from build123d import *

# Parameters (mm, degrees)
SKETCH1_W               = 82
SKETCH1_H               = 46
BOSS_EXTRUDE1_DEPTH     = 25
CUT_EXTRUDE1_REACH      = 70.629
SKETCH2_W               = 76
SKETCH2_H               = 40
CUT_EXTRUDE2_DEPTH      = 89.758098222
CUT_EXTRUDE2_DEPTH_BACK = 89.758098222
SKETCH4_W               = 50
SKETCH4_H               = 3
BOSS_EXTRUDE2_DEPTH     = 71
CUT_EXTRUDE3_REACH      = 124.548
SKETCH5_R               = 1.75
SKETCH7_W               = 16
SKETCH7_H               = 3
BOSS_EXTRUDE4_DEPTH     = 71
SKETCH8_W               = 50
SKETCH8_H               = 46
BOSS_EXTRUDE5_DEPTH     = 3
CUT_EXTRUDE4_DEPTH      = 127.356638132
CUT_EXTRUDE4_DEPTH_BACK = 3
CUT_EXTRUDE5_REACH      = 128.357
SKETCH10_W              = 11
SKETCH10_H              = 5
CUT_EXTRUDE6_REACH      = 128.357
SKETCH11_R              = 1.5
SKETCH12_R              = 15
BOSS_EXTRUDE6_DEPTH     = 30
SKETCH13_R              = 12.5
CUT_EXTRUDE7_DEPTH      = 190.076704012
SKETCH14_W              = 2
SKETCH14_H              = 10.8
SKETCH14_H_2            = 13
BOSS_EXTRUDE7_DEPTH     = 68
CUT_EXTRUDE8_REACH      = 189.343
SKETCH15_R              = 2


with BuildPart() as part:
    # Sketch1 → Boss-Extrude1 (new, symmetric)
    with BuildSketch(Plane.XY):
        Rectangle(SKETCH1_W, SKETCH1_H)
    extrude(amount=BOSS_EXTRUDE1_DEPTH, both=True)

    # Sketch2 → Cut-Extrude1 (cut, up to next)
    with BuildSketch(Plane.XY.offset(25), mode=Mode.PRIVATE) as cut_extrude1_sk1:
        Rectangle(SKETCH2_W, SKETCH2_H)
    cut_extrude1_tool1 = extrude(cut_extrude1_sk1.sketch, amount=-CUT_EXTRUDE1_REACH, mode=Mode.PRIVATE) & part.part
    add(cut_extrude1_tool1.solids().sort_by_distance((0, 0, 25))[0], mode=Mode.SUBTRACT)

    # Sketch3 → Cut-Extrude2 (cut, two sides: drawn at the far end of the back side and taken through both)
    with BuildSketch(Plane.ZY.offset(41).offset(-CUT_EXTRUDE2_DEPTH_BACK)):
        Polygon((-18, 16), (-18, 20), (18, 20), (18, 16), (22, 16), (22, -16), (18, -16), (18, -20), (-18, -20), (-18, -16), (-22, -16), (-22, 16), align=None)
    extrude(amount=CUT_EXTRUDE2_DEPTH + CUT_EXTRUDE2_DEPTH_BACK, mode=Mode.SUBTRACT)

    # Sketch4 → Boss-Extrude2 (add)
    with BuildSketch(Plane(origin=(41, 0, 0), x_dir=(0, 0, -1), z_dir=(1, 0, 0))):
        with Locations((0, -21.5)):
            Rectangle(SKETCH4_W, SKETCH4_H)
    boss_extrude2 = extrude(amount=BOSS_EXTRUDE2_DEPTH)

    # Sketch5 → Cut-Extrude3 (cut, up to next)
    with BuildSketch(Plane(origin=(0, -20, 0), x_dir=(1, 0, 0), z_dir=(0, 1, 0)), mode=Mode.PRIVATE) as cut_extrude3_sk1:
        with Locations(Location((103.1, 20.1, 0), (0, 0, 270))):
            Circle(SKETCH5_R)
    cut_extrude3_tool1 = extrude(cut_extrude3_sk1.sketch, amount=-CUT_EXTRUDE3_REACH, mode=Mode.PRIVATE) & part.part
    # Sketch5 → Cut-Extrude3 (cut, up to next)
    with BuildSketch(Plane(origin=(0, -20, 0), x_dir=(1, 0, 0), z_dir=(0, 1, 0)), mode=Mode.PRIVATE) as cut_extrude3_sk2:
        with Locations(Location((103, -20, 0), (0, 0, 270))):
            Circle(SKETCH5_R)
    cut_extrude3_tool2 = extrude(cut_extrude3_sk2.sketch, amount=-CUT_EXTRUDE3_REACH, mode=Mode.PRIVATE) & part.part
    # Sketch5 → Cut-Extrude3 (cut, up to next)
    with BuildSketch(Plane(origin=(0, -20, 0), x_dir=(1, 0, 0), z_dir=(0, 1, 0)), mode=Mode.PRIVATE) as cut_extrude3_sk3:
        with Locations(Location((50, 20.1, 0), (0, 0, 270))):
            Circle(SKETCH5_R)
    cut_extrude3_tool3 = extrude(cut_extrude3_sk3.sketch, amount=-CUT_EXTRUDE3_REACH, mode=Mode.PRIVATE) & part.part
    # Sketch5 → Cut-Extrude3 (cut, up to next)
    with BuildSketch(Plane(origin=(0, -20, 0), x_dir=(1, 0, 0), z_dir=(0, 1, 0)), mode=Mode.PRIVATE) as cut_extrude3_sk4:
        with Locations(Location((50, -20, 0), (0, 0, 270))):
            Circle(SKETCH5_R)
    cut_extrude3_tool4 = extrude(cut_extrude3_sk4.sketch, amount=-CUT_EXTRUDE3_REACH, mode=Mode.PRIVATE) & part.part
    cut_extrude3_1 = cut_extrude3_tool1.solids().sort_by_distance((103.1, -20, -20.1))[0]
    add(cut_extrude3_1, mode=Mode.SUBTRACT)
    cut_extrude3_2 = cut_extrude3_tool2.solids().sort_by_distance((103, -20, 20))[0]
    add(cut_extrude3_2, mode=Mode.SUBTRACT)
    cut_extrude3_3 = cut_extrude3_tool3.solids().sort_by_distance((50, -20, -20.1))[0]
    add(cut_extrude3_3, mode=Mode.SUBTRACT)
    cut_extrude3_4 = cut_extrude3_tool4.solids().sort_by_distance((50, -20, 20))[0]
    add(cut_extrude3_4, mode=Mode.SUBTRACT)
    cut_extrude3 = cut_extrude3_1 + cut_extrude3_2 + cut_extrude3_3 + cut_extrude3_4  # Cut-Extrude3 as one shape, for the pattern or mirror that repeats it

    # Sketch7 → Boss-Extrude4 (add)
    with BuildSketch(Plane(origin=(41, 0, 0), x_dir=(0, 0, -1), z_dir=(1, 0, 0))):
        with Locations((0, 21.5)):
            Rectangle(SKETCH7_W, SKETCH7_H)
    boss_extrude4 = extrude(amount=BOSS_EXTRUDE4_DEPTH)

    # Sketch8 → Boss-Extrude5 (add)
    with BuildSketch(Plane(origin=(112, 0, 0), x_dir=(0, 0, -1), z_dir=(1, 0, 0))):
        Rectangle(SKETCH8_W, SKETCH8_H)
    extrude(amount=BOSS_EXTRUDE5_DEPTH)

    # Sketch9 → Cut-Extrude4 (cut, two sides: drawn at the far end of the back side and taken through both)
    with BuildSketch(Plane(origin=(0, 23, 0), x_dir=(1, 0, 0), z_dir=(0, 1, 0)).offset(-CUT_EXTRUDE4_DEPTH_BACK)):
        Polygon((105, -317.365996733), (105, -8), (105, -3), (94, -3), (94, -8), (94, -317.365996733), (94, -936.097990199), (105, -936.097990199), align=None)
    extrude(amount=CUT_EXTRUDE4_DEPTH + CUT_EXTRUDE4_DEPTH_BACK, mode=Mode.SUBTRACT)

    # Sketch10 → Cut-Extrude5 (cut, up to next)
    with BuildSketch(Plane(origin=(0, 23, 0), x_dir=(1, 0, 0), z_dir=(0, 1, 0)), mode=Mode.PRIVATE) as cut_extrude5_sk1:
        with Locations((53.5, -5.5)):
            Rectangle(SKETCH10_W, SKETCH10_H)
    cut_extrude5_tool1 = extrude(cut_extrude5_sk1.sketch, amount=-CUT_EXTRUDE5_REACH, mode=Mode.PRIVATE) & part.part
    add(cut_extrude5_tool1.solids().sort_by_distance((53.5, 23, 5.5))[0], mode=Mode.SUBTRACT)

    # Sketch11 → Cut-Extrude6 (cut, up to next)
    with BuildSketch(Plane(origin=(0, 23, 0), x_dir=(1, 0, 0), z_dir=(0, 1, 0)), mode=Mode.PRIVATE) as cut_extrude6_sk1:
        with Locations(Location((45.5, -5.5, 0), (0, 0, 270))):
            Circle(SKETCH11_R)
    cut_extrude6_tool1 = extrude(cut_extrude6_sk1.sketch, amount=-CUT_EXTRUDE6_REACH, mode=Mode.PRIVATE) & part.part
    # Sketch11 → Cut-Extrude6 (cut, up to next)
    with BuildSketch(Plane(origin=(0, 23, 0), x_dir=(1, 0, 0), z_dir=(0, 1, 0)), mode=Mode.PRIVATE) as cut_extrude6_sk2:
        with Locations(Location((61.5, -5.5, 0), (0, 0, 270))):
            Circle(SKETCH11_R)
    cut_extrude6_tool2 = extrude(cut_extrude6_sk2.sketch, amount=-CUT_EXTRUDE6_REACH, mode=Mode.PRIVATE) & part.part
    # Sketch11 → Cut-Extrude6 (cut, up to next)
    with BuildSketch(Plane(origin=(0, 23, 0), x_dir=(1, 0, 0), z_dir=(0, 1, 0)), mode=Mode.PRIVATE) as cut_extrude6_sk3:
        with Locations(Location((91.5, -5.5, 0), (0, 0, 270))):
            Circle(SKETCH11_R)
    cut_extrude6_tool3 = extrude(cut_extrude6_sk3.sketch, amount=-CUT_EXTRUDE6_REACH, mode=Mode.PRIVATE) & part.part
    # Sketch11 → Cut-Extrude6 (cut, up to next)
    with BuildSketch(Plane(origin=(0, 23, 0), x_dir=(1, 0, 0), z_dir=(0, 1, 0)), mode=Mode.PRIVATE) as cut_extrude6_sk4:
        with Locations(Location((107.5, -5.5, 0), (0, 0, 270))):
            Circle(SKETCH11_R)
    cut_extrude6_tool4 = extrude(cut_extrude6_sk4.sketch, amount=-CUT_EXTRUDE6_REACH, mode=Mode.PRIVATE) & part.part
    add(cut_extrude6_tool1.solids().sort_by_distance((45.5, 23, 5.5))[0], mode=Mode.SUBTRACT)
    add(cut_extrude6_tool2.solids().sort_by_distance((61.5, 23, 5.5))[0], mode=Mode.SUBTRACT)
    add(cut_extrude6_tool3.solids().sort_by_distance((91.5, 23, 5.5))[0], mode=Mode.SUBTRACT)
    add(cut_extrude6_tool4.solids().sort_by_distance((107.5, 23, 5.5))[0], mode=Mode.SUBTRACT)

    # Sketch12 → Boss-Extrude6 (add)
    with BuildSketch(Plane(origin=(115, 0, 0), x_dir=(0, 0, -1), z_dir=(1, 0, 0))):
        with Locations((10, 0)):
            Circle(SKETCH12_R)
    extrude(amount=BOSS_EXTRUDE6_DEPTH)

    # Sketch13 → Cut-Extrude7 (cut, through all)
    with BuildSketch(Plane(origin=(145, 0, 0), x_dir=(0, 0, -1), z_dir=(1, 0, 0))):
        with Locations((10, 0)):
            Circle(SKETCH13_R)
    extrude(amount=-CUT_EXTRUDE7_DEPTH, mode=Mode.SUBTRACT)

    # Sketch14 → Boss-Extrude7 (add)
    with BuildSketch(Plane(origin=(115, 0, 0), x_dir=(0, 0, -1), z_dir=(1, 0, 0))):
        with Locations((-3.7, 17.6)):
            Rectangle(SKETCH14_W, SKETCH14_H)
        with Locations((-3.7, -22.5)):
            Rectangle(SKETCH14_W, SKETCH14_H_2)
    extrude(amount=BOSS_EXTRUDE7_DEPTH)

    # Sketch15 → Cut-Extrude8 (cut, up to next)
    with BuildSketch(Plane(origin=(0, 0, 2.7), x_dir=(-1, 0, 0), z_dir=(0, 0, -1)), mode=Mode.PRIVATE) as cut_extrude8_sk1:
        with Locations(Location((-180, -24.8, 0), (0, 0, 90))):
            Circle(SKETCH15_R)
    cut_extrude8_tool1 = extrude(cut_extrude8_sk1.sketch, amount=-CUT_EXTRUDE8_REACH, mode=Mode.PRIVATE) & part.part
    # Sketch15 → Cut-Extrude8 (cut, up to next)
    with BuildSketch(Plane(origin=(0, 0, 2.7), x_dir=(-1, 0, 0), z_dir=(0, 0, -1)), mode=Mode.PRIVATE) as cut_extrude8_sk2:
        with Locations(Location((-160, -24.8, 0), (0, 0, 90))):
            Circle(SKETCH15_R)
    cut_extrude8_tool2 = extrude(cut_extrude8_sk2.sketch, amount=-CUT_EXTRUDE8_REACH, mode=Mode.PRIVATE) & part.part
    # Sketch15 → Cut-Extrude8 (cut, up to next)
    with BuildSketch(Plane(origin=(0, 0, 2.7), x_dir=(-1, 0, 0), z_dir=(0, 0, -1)), mode=Mode.PRIVATE) as cut_extrude8_sk3:
        with Locations(Location((-160, 17.2, 0), (0, 0, 90))):
            Circle(SKETCH15_R)
    cut_extrude8_tool3 = extrude(cut_extrude8_sk3.sketch, amount=-CUT_EXTRUDE8_REACH, mode=Mode.PRIVATE) & part.part
    # Sketch15 → Cut-Extrude8 (cut, up to next)
    with BuildSketch(Plane(origin=(0, 0, 2.7), x_dir=(-1, 0, 0), z_dir=(0, 0, -1)), mode=Mode.PRIVATE) as cut_extrude8_sk4:
        with Locations(Location((-180, 17.2, 0), (0, 0, 90))):
            Circle(SKETCH15_R)
    cut_extrude8_tool4 = extrude(cut_extrude8_sk4.sketch, amount=-CUT_EXTRUDE8_REACH, mode=Mode.PRIVATE) & part.part
    add(cut_extrude8_tool1.solids().sort_by_distance((180, -24.8, 2.7))[0], mode=Mode.SUBTRACT)
    add(cut_extrude8_tool2.solids().sort_by_distance((160, -24.8, 2.7))[0], mode=Mode.SUBTRACT)
    add(cut_extrude8_tool3.solids().sort_by_distance((160, 17.2, 2.7))[0], mode=Mode.SUBTRACT)
    add(cut_extrude8_tool4.solids().sort_by_distance((180, 17.2, 2.7))[0], mode=Mode.SUBTRACT)

    # Mirror1: Boss-Extrude2, Cut-Extrude3, Boss-Extrude4 across plane
    add(boss_extrude2.mirror(Plane(origin=(0, 0, 0), x_dir=(0, 0, 1), z_dir=(1, 0, 0))))
    add(cut_extrude3.mirror(Plane(origin=(0, 0, 0), x_dir=(0, 0, 1), z_dir=(1, 0, 0))), mode=Mode.SUBTRACT)
    add(boss_extrude4.mirror(Plane(origin=(0, 0, 0), x_dir=(0, 0, 1), z_dir=(1, 0, 0))))


solid = part.part
Design review of the part built by this model. Coordinates are the model's own, in mm. A direction names the side the tool comes from. Coordinates: 2 decimals unless noted, no trailing zeros. Loops run counter-clockwise (first coordinate to the right, second up) from the corner with the lowest first, then second, coordinate; pieces in that order, holes last. Notation, with made-up numbers: (14, 30.25) - (71, 30.25) arc R19 cw to (71, 35.25) - close; hole circle Ø5 at (43.25, -0.75). An arc over 180 degrees is marked (long way). Use CSV: the item, a comma, the result in double quotes. Start each with the question number.
1. Add section D-D on x = 77. Give the boundary of the cut face in (y, z), plus the area to 3 significant figures.
2. Add section A-A on x = 7. Give the boundary of the cut face in (y, z).
3. Mouldability with a two-part tool opening along X and no side actions: class faces 6 (the flat face through (41, 5, -23)), 7 (the flat face through (149, 18, 4.7)), 8 (the flat face through (-41, 4.6, 22.2)) as released by +X, released by -X, zero draft, split by the parting line, or undercut.
4. Clearance check with flat-ended pins moving along their axes: pin 1 (6 mm diameter, centred on x = 131.5, y = -13.5, fed in from +Z); pin 2 (4 mm diameter, centred on x = -8, z = -19.5, fed in from -Y); pin 3 (2 mm diameter, centred on y = -19, z = 10.5, fed in from +X); pin 4 (4 mm diameter, centred on x = 107.5, z = 5.5, fed in from +Y). State where each tip first meets the part, or that it passes through.
5. Add section C-C on y = 8. Give the boundary of the cut face in (x, z).
6. To check wall thickness, follow probe 1 along Y at (x, z) = (160, 3.75); probe 2 along X at (y, z) = (-20.65, -20.1); probe 3 along Z at (x, y) = (103, -22). State the ranges of each line that lie inside material, in increasing order.
7. For faces 1 (the flat face through (-41, 5, -23)), 2 (the flat face through (149, -23, 4.7)), 3 (the flat face through (-6, -21, 25)), 4 (the flat face through (41, 4.6, 22.2)), 5 (the flat face through (38, 0, -23)), list the 3-axis set-ups (+Z, -Z, +X, -X, +Y, -Y) from which the entire face can be reached by the end or side of a thin tool; tool diameter is ignored.
8. Add section B-B on z = -3.5. Give the boundary of the cut face in (x, y).
Resolved:
1,outline,"(-23, -25) - (-20, -25) - (-20, 25) - (-23, 25) - close; (20, -8) - (23, -8) - (23, 8) - (20, 8) - close"
1,area,"198 mm2"
2,outline,"(-23, -25) - (-20, -25) - (-20, 25) - (-23, 25) - close; (20, -25) - (23, -25) - (23, 25) - (20, 25) - close"
3,face 6,"undercut"
3,face 7,"zero draft"
3,face 8,"released by -X"
4,pin 1,"z = 4.7"
4,pin 2,"y = -23"
4,pin 3,"x = 115"
4,pin 4,"y = 23"
5,outline,"(-41, -25) - (-38, -25) - (-38, -22) - (-41, -22) - close; (-41, 22) - (-38, 22) - (-38, 25) - (-41, 25) - close; (38, -25) - (41, -25) - (41, -22) - (38, -22) - close; (38, 22) - (41, 22) - (41, 25) - (38, 25) - close; (112, -25) - (115, -25) - (115, -22.69) - (145, -22.69) - (145, -19.6) - (112, -19.6) - close; (112, -0.4) - (145, -0.4) - (145, 2.69) - (115, 2.69) - (115, 25) - (112, 25) - close"
6,probe 1,"-29 to -26.8, -22.8 to -16, 12.2 to 15.2, 19.2 to 23"
6,probe 2,"-112 to -104.85, -101.35 to -51.75, -48.25 to 48.25, 51.75 to 101.35, 104.85 to 115"
6,probe 3,"-25 to -21.85, -18.35 to 18.25, 21.75 to 25"
7,face 1,"-Z, -X, +Y"
7,face 2,"+Z, +X, -Y"
7,face 3,"+Z, +X, -X, +Y, -Y"
7,face 4,"+Z, +Y"
7,face 5,"+Z, -Z"
8,outline,"(-112, -23) - (115, -23) - (115, -13.52) - (145, -13.52) - (145, -10.68) - (112, -10.68) - (112, -20) - (-112, -20) - close; (-112, 20) - (112, 20) - (112, 10.68) - (145, 10.68) - (145, 13.52) - (115, 13.52) - (115, 23) - (-112, 23) - close"
